```python
from build123d import *

# Parameters (mm, degrees)
SKETCH1_R           = 13.5
SKETCH1_R_2         = 18.5
BOSS_EXTRUDE1_DEPTH = 100
CUT_EXTRUDE1_DEPTH  = 11.5
SKETCH4_R           = 0.7
CUT_EXTRUDE2_DEPTH  = 10
SKETCH5_W           = 127
SKETCH5_H           = 47.647991038
CUT_EXTRUDE3_DEPTH  = 40
SKETCH6_R           = 7.5
SKETCH6_W           = 16
SKETCH6_H           = 40
CUT_EXTRUDE4_DEPTH  = 92.5
SKETCH10_R          = 10.5
CUT_EXTRUDE5_DEPTH  = 25.5
SKETCH11_W          = 135
SKETCH11_H          = 35
BOSS_EXTRUDE2_DEPTH = 10
SKETCH12_W          = 31.059733337
SKETCH12_H          = 3
CUT_EXTRUDE6_DEPTH  = 125
SKETCH13_R          = 5
CUT_EXTRUDE8_DEPTH  = 10
SKETCH14_R          = 10
CUT_EXTRUDE9_DEPTH  = 2


with BuildPart() as part:
    # Sketch1 → Boss-Extrude1 (new body)
    with BuildSketch(Plane(origin=(0, 0, 0), x_dir=(1, 0, 0), z_dir=(0, 1, 0))):
        Polygon((-82.5, 0), (-82.5, -35), (52.5, -35), (52.5, 0), (52.5, 45), (-82.5, 45), align=None)
        with Locations(Location((-60, 22.5, 0), (0, 0, 270))):
            Circle(SKETCH1_R, mode=Mode.SUBTRACT)
        with Locations(Location((-15, 22.5, 0), (0, 0, 270))):
            Circle(SKETCH1_R_2, mode=Mode.SUBTRACT)
        with Locations(Location((30, 22.5, 0), (0, 0, 270))):
            Circle(SKETCH1_R, mode=Mode.SUBTRACT)
    extrude(amount=BOSS_EXTRUDE1_DEPTH)

    # Sketch3 → Cut-Extrude1 (cut)
    with BuildSketch(Plane.XZ):
        with BuildLine():
            Line((-32.158714626, -40.681818182), (2.158714626, -40.681818182))
            ThreePointArc((2.158714626, -40.681818182), (10, -22.5), (2.158714626, -4.318181818))
            Line((2.158714626, -4.318181818), (-32.158714626, -4.318181818))
            ThreePointArc((-32.158714626, -4.318181818), (-40, -22.5), (-32.158714626, -40.681818182))
        make_face()
    extrude(amount=-CUT_EXTRUDE1_DEPTH, mode=Mode.SUBTRACT)

    # Sketch4 → Cut-Extrude2 (cut)
    with BuildSketch(Plane.XZ.offset(-11.5)):
        with Locations(Location((-36.25, -22.5, 0), (0, 0, 270))):
            Circle(SKETCH4_R)
        with Locations(Location((-30.0260191, -7.4739809, 0), (0, 0, 270))):
            Circle(SKETCH4_R)
        with Locations(Location((0.0260191, -7.4739809, 0), (0, 0, 270))):
            Circle(SKETCH4_R)
        with Locations(Location((6.25, -22.5, 0), (0, 0, 270))):
            Circle(SKETCH4_R)
        with Locations(Location((0.0260191, -37.5260191, 0), (0, 0, 270))):
            Circle(SKETCH4_R)
        with Locations(Location((-30.0260191, -37.5260191, 0), (0, 0, 270))):
            Circle(SKETCH4_R)
    extrude(amount=-CUT_EXTRUDE2_DEPTH, mode=Mode.SUBTRACT)

    # Sketch5 → Cut-Extrude3 (cut)
    with BuildSketch(Plane(origin=(0, 100, 0), x_dir=(1, 0, 0), z_dir=(0, 1, 0))):
        with Locations((-15, 23.823995519)):
            Rectangle(SKETCH5_W, SKETCH5_H)
    extrude(amount=-CUT_EXTRUDE3_DEPTH, mode=Mode.SUBTRACT)

    # Sketch6 → Cut-Extrude4 (cut)
    with BuildSketch(Plane.ZY.offset(82.5)):
        with Locations((17.5, 85)):
            Circle(SKETCH6_R)
        with Locations(Location((17.5, 15, 0), (0, 0, 180))):
            Circle(SKETCH6_R)
        with Locations((17.5, 50)):
            Rectangle(SKETCH6_W, SKETCH6_H)
    extrude(amount=-CUT_EXTRUDE4_DEPTH, mode=Mode.SUBTRACT)

    # Sketch10 → Cut-Extrude5 (cut)
    with BuildSketch(Plane.XY.offset(35)):
        with Locations((-15, 49.733985677)):
            Circle(SKETCH10_R)
    extrude(amount=-CUT_EXTRUDE5_DEPTH, mode=Mode.SUBTRACT)

    # Sketch11 → Boss-Extrude2 (add)
    with BuildSketch(Plane.XZ):
        with Locations((-15, 17.5)):
            Rectangle(SKETCH11_W, SKETCH11_H)
    extrude(amount=BOSS_EXTRUDE2_DEPTH)

    # Sketch12 → Cut-Extrude6 (cut)
    with BuildSketch(Plane.ZY.offset(82.5)):
        with Locations((20.529866669, -5)):
            Rectangle(SKETCH12_W, SKETCH12_H)
    extrude(amount=-CUT_EXTRUDE6_DEPTH, mode=Mode.SUBTRACT)

    # Sketch13 → Cut-Extrude8 (cut)
    with BuildSketch(Plane.XZ.offset(10)):
        with Locations(Location((-62.5, 17.5, 0), (0, 0, 270))):
            Circle(SKETCH13_R)
        with Locations(Location((32.5, 17.5, 0), (0, 0, 270))):
            Circle(SKETCH13_R)
        with Locations(Location((-15, 17.5, 0), (0, 0, 270))):
            Circle(SKETCH13_R)
    extrude(amount=-CUT_EXTRUDE8_DEPTH, mode=Mode.SUBTRACT)

    # Sketch14 → Cut-Extrude9 (cut)
    with BuildSketch(Plane.XZ.offset(10)):
        with Locations(Location((-62.5, 17.5, 0), (0, 0, 270))):
            Circle(SKETCH14_R)
        with Locations(Location((-15, 17.5, 0), (0, 0, 270))):
            Circle(SKETCH14_R)
        with Locations(Location((32.5, 17.5, 0), (0, 0, 270))):
            Circle(SKETCH14_R)
    extrude(amount=-CUT_EXTRUDE9_DEPTH, mode=Mode.SUBTRACT)


solid = part.part
```
Build history of the part. All positions in model axes, mm. A direction names the side the tool comes from. Round coordinates to 2 decimals unless told otherwise and drop trailing zeros. Write each loop counter-clockwise with the first axis right and the second up, starting at its lowest first coordinate (ties: lowest second). Pieces come first, ordered by that corner, then holes. Notation, with made-up numbers: (4, -25) - (17, -25) arc R19 cw to (17, -18) - close; hole circle Ø4 at (-39.75, 2). An arc over 180 degrees is marked (long way). Write each question's results on one line, items separated by ' | '. Start each with the question number.
Item 1: Saw through at B-B (x = -49.5). Write the cut outline in (y, z), and give its area (3 significant figures).
Item 2: Which spindle directions (+Z, -Z, +X, -X, +Y, -Y) get a long thin tool onto all of the face, cutting with end or side? Do faces 1 (the face through (-16, 0, -43)), 2 (the face through (-57.543, -7.26, 18.151)), 3 (the face through (10, 85, 17)), 4 (the face through (-21, -5, 5)). Say none if no direction does.
Item 3: Saw through at D-D (x = 32.5). Write the cut outline in (y, z).
Item 4: Mould opens along X. For faces 5 (the face through (-21, -6.5, 20)), 6 (the face through (42.5, -5, 20)), 7 (the face through (-19.88, -7.26, 18.58)) say: pulls with the +X half, pulls with the -X half, needs draft (parallel to the pull), parting line crosses it, or undercut.
Item 5: Saw through at A-A (y = 26). Write the cut outline in (x, z).
Item 6: Wall check: L1, parallel to X at y = -9, z = 17; L2, parallel to X at y = 16, z = -22.5; L3, parallel to Y at x = -22, z = 17.5. Give the ranges that are in metal, low to high. Write a range as [from, to].
Item 7: Drop flat-ended pins along their axis: P1, Ø12, axis at y = 14, z = 17, coming from the -X side; P2, Ø6, axis at x = -15, z = 20.5, coming from the -Y side; P3, Ø8, axis at x = -62, y = 76.5, coming from the -Z side. Give the stop position or say it passes through.
Item 8: Saw through at C-C (y = 48). Write the cut outline in (x, z), and give its area (3 significant figures).
Results are:
1) outline: (-10, 0) - (0, 0) - (0, -14.01) - (60, -14.01) - (60, 0) - (100, 0) - (100, 35) - (-3.5, 35) - (-3.5, 5) - (-6.5, 5) - (-6.5, 35) - (-10, 35) - close; (0, -45) - (60, -45) - (60, -30.99) - (0, -30.99) - close; hole circle Ø15 at (15, 17.5); hole (30, 9.5) - (70, 9.5) - (70, 25.5) - (30, 25.5) - close; hole circle Ø15 at (85, 17.5) | area: 4,450 mm²
2) face 1: -Z, +X, -X, -Y | face 2: -Y | face 3: -X | face 4: +Z, -X
3) outline: (-10, 0) - (0, 0) - (0, -9.23) - (60, -9.23) - (60, 0) - (100, 0) - (100, 35) - (-3.5, 35) - (-3.5, 22.5) - (0, 22.5) - (0, 12.5) - (-3.5, 12.5) - (-3.5, 5) - (-6.5, 5) - (-6.5, 12.5) - (-8, 12.5) - (-8, 7.5) - (-10, 7.5) - close; (-10, 27.5) - (-8, 27.5) - (-8, 22.5) - (-6.5, 22.5) - (-6.5, 35) - (-10, 35) - close; (0, -45) - (60, -45) - (60, -35.77) - (0, -35.77) - close
4) face 5: needs draft | face 6: pulls with the -X half | face 7: undercut
5) outline: (-82.5, -45) - (52.5, -45) - (52.5, 35) - (-82.5, 35) - close; hole circle Ø27 at (-60, -22.5); hole circle Ø37 at (-15, -22.5); hole circle Ø27 at (30, -22.5)
6) L1: x = [-82.5, -72.49], [-52.51, -24.99], [-5.01, 22.51], [42.49, 52.5] | L2: x = [-82.5, -73.5], [-46.5, -36.95], [-35.55, -33.5], [3.5, 5.55], [6.95, 16.5], [43.5, 52.5] | L3: y = [-8, -6.5], [-3.5, 7.5], [22.5, 30], [70, 77.5], [92.5, 100]
7) P1: stops at x = 10 | P2: stops at y = -8 | P3: stops at z = 0
8) outline: (-82.5, -45) - (52.5, -45) - (52.5, 35) - (-4.64, 35) - (-4.64, 25.5) - (10, 25.5) - (10, 9.5) - (-82.5, 9.5) - close; (-82.5, 25.5) - (-25.36, 25.5) - (-25.36, 35) - (-82.5, 35) - close; hole circle Ø27 at (-60, -22.5); hole circle Ø37 at (-15, -22.5); hole circle Ø27 at (30, -22.5) | area: 6,900 mm²
